from build123d import *

# Parameters (mm, degrees)
SKETCH1_W            = 62.5
SKETCH1_H            = 25
SKETCH1_R            = 2.25
BASE_FLANGE1_DEPTH   = 0.4
EDGE_FLANGE1_START   = 37.3
EDGE_FLANGE1_DEPTH   = 25.2
EDGE_FLANGE1_2_DEPTH = 0.2
EDGE_FLANGE1_START_2 = 37.5
EDGE_FLANGE1_3_DEPTH = 25
EDGE_FLANGE2_DEPTH   = 25


# Read off the part's stored shape, not the designer's step: Edge-Flange1
# Sheet-metal steps are written as plain solids
with BuildPart() as part:
    # Sketch1 → Base-Flange1 (new body)
    with BuildSketch(Plane.XY):
        with Locations((31.25, 12.5)):
            Rectangle(SKETCH1_W, SKETCH1_H)
        with Locations((12.5, 12.5)):
            Circle(SKETCH1_R, mode=Mode.SUBTRACT)
        with Locations((37.5, 12.5)):
            Circle(SKETCH1_R, mode=Mode.SUBTRACT)
    extrude(amount=-BASE_FLANGE1_DEPTH)

    # Edge-Flange1 outline → Edge-Flange1 (cut)
    with BuildSketch(Plane.YZ.offset(EDGE_FLANGE1_START)):
        with BuildLine():
            Line((0, -0.4), (0.887156424, -0.4))
            ThreePointArc((0.887156424, -0.4), (0.410375552, -0.295165264), (0.021546812, 0))
            Line((0.021546812, 0), (0, 0))
            Line((0, 0), (0, -0.4))
        make_face()
    extrude(amount=EDGE_FLANGE1_DEPTH, mode=Mode.SUBTRACT)

    # Edge-Flange1 2 outline → Edge-Flange1 2 (cut)
    with BuildSketch(Plane.YZ.offset(EDGE_FLANGE1_START)):
        with BuildLine():
            Line((1.087156424, -0.4), (1.087156424, 0))
            Line((1.087156424, 0), (0.021546812, 0))
            ThreePointArc((0.021546812, 0), (0.410375552, -0.295165264), (0.887156424, -0.4))
            Line((0.887156424, -0.4), (1.087156424, -0.4))
        make_face()
    extrude(amount=EDGE_FLANGE1_2_DEPTH, mode=Mode.SUBTRACT)

    # Edge-Flange1 3 outline → Edge-Flange1 3 (add)
    with BuildSketch(Plane.YZ.offset(EDGE_FLANGE1_START_2)):
        with BuildLine():
            Line((0.021546812, 0), (0.887156424, 0))
            ThreePointArc((0.887156424, 0), (0.518856424, 0.098685688), (0.249242111, 0.3683))
            Line((0.249242111, 0.3683), (-3.422649731, 6.72820323))
            Line((-3.422649731, 6.72820323), (-3.769059892, 6.52820323))
            Line((-3.769059892, 6.52820323), (-0.09716805, 0.1683))
            ThreePointArc((-0.09716805, 0.1683), (-0.041630555, 0.081455507), (0.021546812, 0))
        make_face()
    extrude(amount=EDGE_FLANGE1_3_DEPTH)

    # Edge-Flange2 section (across the edge) → Edge-Flange2 (add)
    with BuildSketch(Plane(origin=(62.5, -3.981697996, 6.89650323), x_dir=(0, 0, -1), z_dir=(-1, 0, 0))):
        with BuildLine():
            Line((-0.4, 0.425276208), (-0.4, 57.769059892))
            Line((-0.4, 57.769059892), (0, 57.769059892))
            Line((0, 57.769059892), (0, 0.425276208))
            ThreePointArc((0, 0.425276208), (0.098685688, 0.056976208), (0.3683, -0.212638104))
            Line((0.3683, -0.212638104), (0.1683, -0.559048266))
            ThreePointArc((0.1683, -0.559048266), (-0.247724474, -0.143023792), (-0.4, 0.425276208))
        make_face()
    extrude(amount=EDGE_FLANGE2_DEPTH)


solid = part.part
Read the model definition and answer for the solid it produces. Units are mm, in the model's axes. A direction names the side the tool comes from. Coordinates: 2 decimals unless noted, no trailing zeros. Write each loop counter-clockwise with the first axis right and the second up, starting at its lowest first coordinate (ties: lowest second). Pieces come first, ordered by that corner, then holes. Notation, with made-up numbers: (-19.75, 54) -> (28.25, 54) arc R12 cw to (28.25, 73) -> close; hole circle Ø9 at (88, 26). An arc over 180 degrees is marked (long way). Return JSON: item names as keys, results as strings.
(1) Which of the six approach directions +Z, -Z, +X, -X, +Y, -Y give full straight-line access (tool end or side, diameter ignored) to faces 1 (the flat face through (50, -33, 6.897)), 2 (the flat face through (49.82, -1.56, 3.5))?
Answers below:
{"face 1": "-Z, +X, -X, -Y", "face 2": "+Z, +X, -X, +Y"}
(2) The part is cut by section A-A on x = 12.5. Give the vertices of the cut face in (y, z).
Answers below:
{"outline": "(0, -0.4) -> (10.25, -0.4) -> (10.25, 0) -> (0, 0) -> close; (14.75, -0.4) -> (25, -0.4) -> (25, 0) -> (14.75, 0) -> close"}
(3) For a pull along X with two mould halves and no side action, classify faces 3 (the flat face through (31, 13, -0.4)), 4 (the flat face through (62.5, -15.4, 7.1)), 5 (the cylindrical face through (38.71, 14.397, -0.197)) as pulls with the +X half, pulls with the -X half, needs draft (parallel to the pull), parting line crosses it, or undercut.
Answers below:
{"face 3": "needs draft", "face 4": "pulls with the +X half", "face 5": "undercut"}
(4) The part is cut by section C-C on x = 56.5. Give the vertices of the cut face in (y, z).
Answers below:
{"outline": "(-61.75, 6.9) -> (-4.41, 6.9) arc R0.74 cw to (-3.77, 6.53) -> (-0.1, 0.17) arc R1.14 ccw to (0.89, -0.4) -> (25, -0.4) -> (25, 0) -> (0.89, 0) arc R0.74 cw to (0.25, 0.37) -> (-3.42, 6.73) arc R1.14 ccw to (-4.41, 7.3) -> (-61.75, 7.3) -> close"}
(5) The part is cut by section D-D on z = 4.25. Give the vertices of the cut face in (x, y).
Answers below:
{"outline": "(37.5, -2.45) -> (62.5, -2.45) -> (62.5, -1.99) -> (37.5, -1.99) -> close"}
(6) The part is cut by section B-B on y = 12.5. Give the vertices of the cut face in (x, z), then the cut area to 3 significant figures.
Answers below:
{"outline": "(0, -0.4) -> (10.25, -0.4) -> (10.25, 0) -> (0, 0) -> close; (14.75, -0.4) -> (35.25, -0.4) -> (35.25, 0) -> (14.75, 0) -> close; (39.75, -0.4) -> (62.5, -0.4) -> (62.5, 0) -> (39.75, 0) -> close", "area": "21.4 mm^2"}
(7) Each of these flat-tipped pins is pushed along its axis until it touches: P1, Ø12.5, axis at x = 50, y = -47.5, coming from the -Z side; P2, Ø4, axis at y = -18.5, z = 5.5, coming from the -X side; P3, Ø10, axis at x = 29, y = -16, coming from the -Z side; P4, Ø7.5, axis at x = 46.5, y = 7, coming from the +Z side. Where does it stop, or does it pass through?
Answers below:
{"P1": "z = 6.9", "P2": "x = 37.5", "P3": "through", "P4": "z = 0"}
(8) Consider line 1 along Y through (x, z) = (12.5, -0.3); line 2 along Z through (x, y) = (45, -33); line 3 along Z through (x, y) = (46, 15.5). Determine where each line is inside the solid, lowest interval first. Write a range as from..to.
Answers below:
{"line 1": "0..10.25, 14.75..25", "line 2": "6.9..7.3", "line 3": "-0.4..0"}
